Work out the finished part from the listing and answer in its coordinate system (mm). Face numbers are marked on the shaded views. A direction names the side the tool comes from. Round coordinates to 2 decimals unless told otherwise and drop trailing zeros. Write each loop counter-clockwise with the first axis right and the second up, starting at its lowest first coordinate (ties: lowest second). Pieces come first, ordered by that corner, then holes. Notation, with made-up numbers: M 65,2.25 L 94,2.25 A19 cw 94,9.25 Z; hole C -29,4 d7. An arc over 180 degrees is marked long. One line per item, written item: value. Start each with the question number.
Q1. Find section B-B (x = -8). Write down the section's boundary in (y, z).
Q2. A tool of negligible diameter and unlimited length cuts with its end or side. For the marked faces 1, 2, 3, 4 and 5, from which of +Z, -Z, +X, -X, +Y, -Y can it reach the whole face along a straight path? Write none if from no direction.
Q3. Consider probe 1 along Y at (x, z) = (-13, 1.5); probe 2 along Y at (x, z) = (-3, 5.25); probe 3 along X at (y, z) = (-7, 4.5). Determine where each line is inside the solid, lowest interval first.
Q4. The mould has two halves that part along X. Classify the marked faces 6, 7, 8 and 9: released by +X, released by -X, zero draft, split by the parting line, or undercut.
Q5. Find section A-A (y = -5.5). Write down the section's boundary in (x, z).
Q6. Given pin 1 Ø3 at (y, z) = (-6.5, 3.5) entering from -X; pin 2 Ø12 at (x, y) = (-6, 39) entering from -Z; pin 3 Ø2 at (x, z) = (-4, 4.5) entering from +Y; pin 4 Ø3 at (x, z) = (-5, 3.5) entering from +Y, each flat-ended and moving along its own axis, determine where each tip first touches the part or whether it passes through.
Q7. Find section D-D (x = 11.5). Write down the section's boundary in (y, z), and give its area (3 significant figures).
Q8. Find section C-C (z = 2.75). Write down the section's boundary in (x, y).
from build123d import *

# Parameters (mm, degrees)
BOSS_EXTRUDE1_DEPTH = 6.35
SKETCH2_W           = 4.4
SKETCH2_H           = 5.72
CUT_EXTRUDE1_DEPTH  = 57.85115788


with BuildPart() as part:
    # Sketch1 → Boss-Extrude1 (new body)
    with BuildSketch(Plane.XY):
        Polygon((-12.346676125, 38.1), (-18.696676125, 38.1), (-18.696676125, 25.4), (-12.346676125, 25.4), (-12.346676125, 19.05), (-18.696676125, 19.05), (-18.696676125, 5.2705), (-12.346676125, 5.2705), (-12.346676125, 9.455763351), (-2.346676125, 9.455763351), (-2.346676125, 5.2705), (-2.346676125, 0), (-12.346676125, 0), (-12.346676125, -15.5875), (29.935330231, -15.5875), (29.935330231, -0.710514446), (-12.346676125, 47.9125), align=None)
    extrude(amount=BOSS_EXTRUDE1_DEPTH)

    # Sketch2 → Cut-Extrude1 (cut, through all)
    with BuildSketch(Plane(origin=(0, 0, 0), x_dir=(-1, 0, 0), z_dir=(0, 0, -1))):
        with Locations((3.796676125, -6.3775)):
            Rectangle(SKETCH2_W, SKETCH2_H)
    extrude(amount=-CUT_EXTRUDE1_DEPTH, mode=Mode.SUBTRACT)


solid = part.part
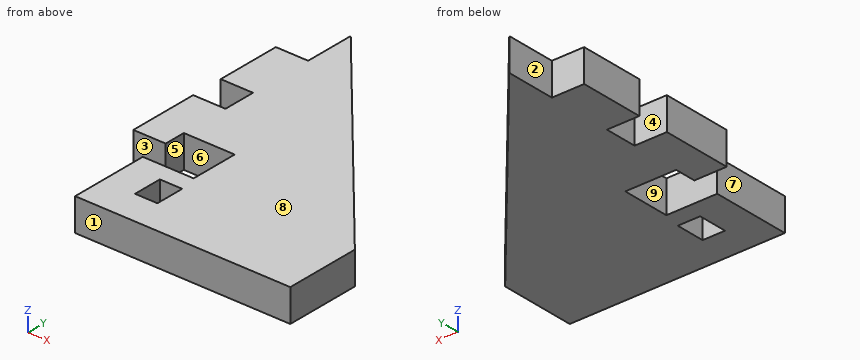
The answers:
1. outline: M -15.59,0 L 0,0 L 0,6.35 L -15.59,6.35 Z; M 9.46,0 L 42.91,0 L 42.91,6.35 L 9.46,6.35 Z
2. face 1: +Z, -Z, +X, -X, -Y
2. face 2: +Z, -Z, -X, +Y
2. face 3: +Z, -Z, -X, -Y
2. face 4: +Z, -Z, -X
2. face 5: +Z, -Z
3. probe 1: 5.27 to 19.05, 25.4 to 38.1
3. probe 2: -15.59 to -9.24, -3.52 to 0, 9.46 to 37.16
3. probe 3: -12.35 to -6, -1.6 to 29.94
4. face 6: undercut
4. face 7: released by -X
4. face 8: zero draft
4. face 9: undercut
5. outline: M -12.35,0 L -6,0 L -6,6.35 L -12.35,6.35 Z; M -1.6,0 L 29.94,0 L 29.94,6.35 L -1.6,6.35 Z
6. pin 1: x = -12.35
6. pin 2: z = 0
6. pin 3: y = 39.46
6. pin 4: y = 41.19
7. outline: M -15.59,0 L 20.49,0 L 20.49,6.35 L -15.59,6.35 Z
7. area: 229 mm2
8. outline: M -18.7,5.27 L -12.35,5.27 L -12.35,9.46 L -2.35,9.46 L -2.35,0 L -12.35,0 L -12.35,-15.59 L 29.94,-15.59 L 29.94,-0.71 L -12.35,47.91 L -12.35,38.1 L -18.7,38.1 L -18.7,25.4 L -12.35,25.4 L -12.35,19.05 L -18.7,19.05 Z; hole M -6,-9.24 L -1.6,-9.24 L -1.6,-3.52 L -6,-3.52 Z
